Drawing for the job (mm, zero at the part's lowest x, y, z). A direction names the side the tool comes from. Round coordinates to 2 decimals unless told otherwise and drop trailing zeros. Loops run counter-clockwise (first coordinate to the right, second up) from the corner with the lowest first, then second, coordinate; pieces in that order, holes last. Notation, with made-up numbers: M 64,-32 L 116,-32 A18 cw 116,1 Z; hole C -25.75,-40 d8. An arc over 180 degrees is marked long. Put each result on its own line as item: value. Start each with the question number.
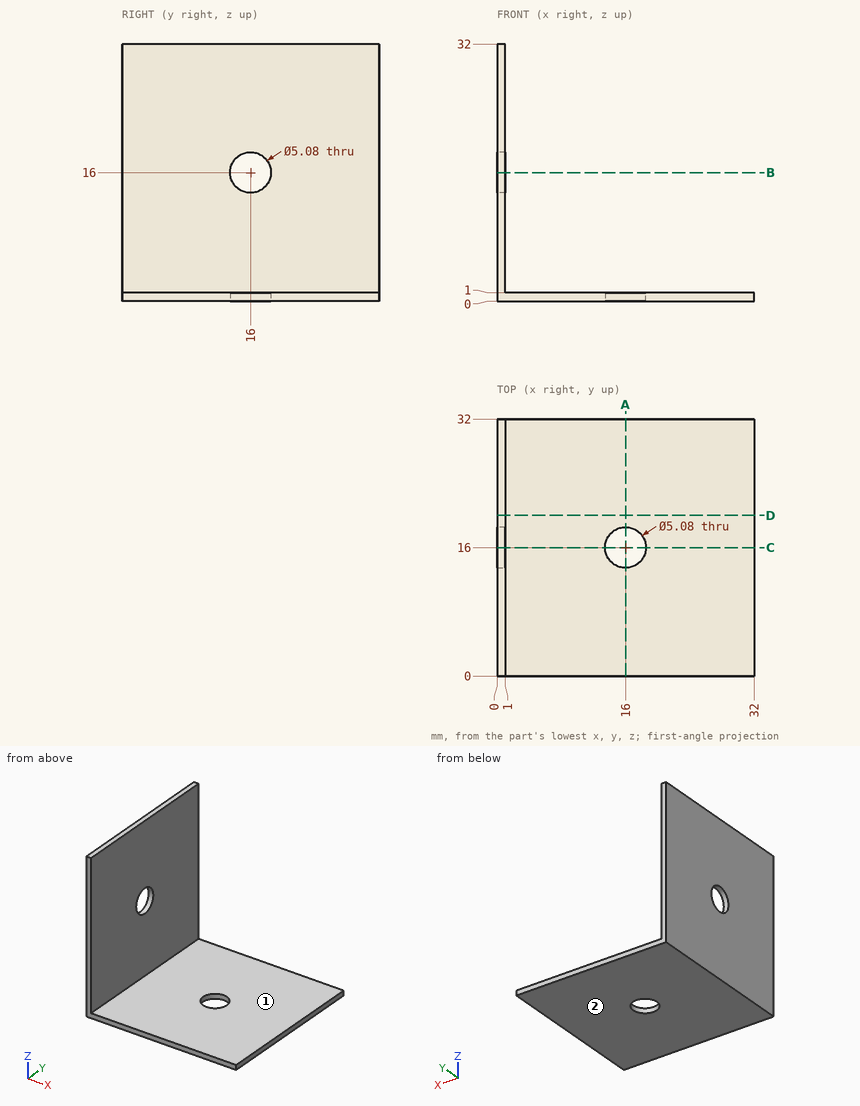
1. Cut at D-D, the plane y = 20. Give the cut face in (x, z), and give its area (3 significant figures).
2. Cut at A-A, the plane x = 16. Give the cut face in (y, z).
3. Cut at B-B, the plane z = 16. Give the cut face in (x, y), and give its area (3 significant figures).
4. Cut at C-C, the plane y = 16. Give the cut face in (x, z), and give its area (3 significant figures).
5. Which spindle directions (+Z, -Z, +X, -X, +Y, -Y) get a long thin tool onto all of the face, cutting with end or side? Do the marked faces 1 and 2. Say none if no direction does.
6. Drop flat-ended pins along their axis: pin 1 (1 mm diameter, centred on x = 3.5, y = 16, fed in from +Z); pin 2 (3 mm diameter, centred on y = 21.5, z = 7.5, fed in from -X); pin 3 (4 mm diameter, centred on y = 16, z = 16, fed in from +X); pin 4 (6 mm diameter, centred on y = 18.5, z = 26, fed in from +X). Give the stop position or say it passes through.
7. Wall check: L1, parallel to X at y = 16, z = 0.5; L2, parallel to Z at x = 25, y = 20.5. Give the ranges that are in metal, low to high.
Results list:
1. outline: M 0,0 L 32,0 L 32,1 L 1,1 L 1,32 L 0,32 Z
1. area: 63.0 mm^2
2. outline: M 0,0 L 13.46,0 L 13.46,1 L 0,1 Z; M 18.54,0 L 32,0 L 32,1 L 18.54,1 Z
3. outline: M 0,0 L 1,0 L 1,13.46 L 0,13.46 Z; M 0,18.54 L 1,18.54 L 1,32 L 0,32 Z
3. area: 26.9 mm^2
4. outline: M 0,0 L 13.46,0 L 13.46,1 L 1,1 L 1,13.46 L 0,13.46 Z; M 0,18.54 L 1,18.54 L 1,32 L 0,32 Z; M 18.54,0 L 32,0 L 32,1 L 18.54,1 Z
4. area: 52.8 mm^2
5. face 1: +Z, +X, +Y, -Y
5. face 2: -Z, +X, -X, +Y, -Y
6. pin 1: stops at z = 1
6. pin 2: stops at x = 0
6. pin 3: passes through
6. pin 4: stops at x = 1
7. L1: x = 0 to 13.46, 18.54 to 32
7. L2: z = 0 to 1
